Geometry: final body of the model. Coordinates: model frame, mm. Face numbers are marked on the shaded views. A direction names the side the tool comes from. Coordinates: 2 decimals unless noted, no trailing zeros. Write each loop counter-clockwise with the first axis right and the second up, starting at its lowest first coordinate (ties: lowest second). Pieces come first, ordered by that corner, then holes.
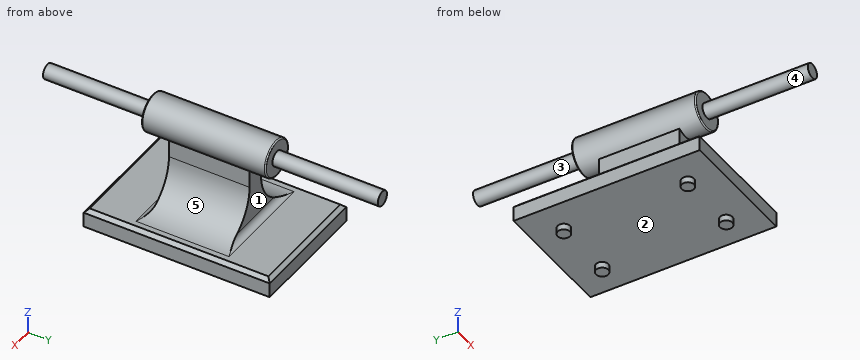
from build123d import *

# Parameters (mm, degrees)
F1_DEPTH  = 75
F2_W      = 15
F2_H      = 65
F3_DEPTH  = 70
F4_R      = 15
F5_DEPTH  = 50
F6_R      = 6
F7_DEPTH  = 85
F8_R      = 6
F9_DEPTH  = 85
F10_R     = 5
F11_DEPTH = 5
F12_R     = 35
F13_R     = 5
F14_SIZE  = 3
F15_R     = 1


with BuildPart() as f1:
    # F0 (on Front) → F1 (new body, symmetric)
    with BuildSketch(Plane.XZ):
        Polygon((50, -7.5), (50, 7.5), (-50, 7.5), (-50, -7.5), (-27.5, -7.5), (27.5, -7.5), align=None)
    extrude(amount=F1_DEPTH, both=True)

    # F2 (on Top) → F3 (join)
    with BuildSketch(Plane.XY):
        Rectangle(F2_W, F2_H)
    extrude(amount=F3_DEPTH)

    # F4 (on Front) → F5 (join, symmetric)
    with BuildSketch(Plane.XZ):
        with Locations((0, 69.991633)):
            Circle(F4_R)
    extrude(amount=F5_DEPTH, both=True)

    # F6 (on face) → F7 (join)
    with BuildSketch(Plane(origin=(0, 50, 0), x_dir=(-1, 0, 0), z_dir=(0, 1, 0))):
        with Locations((0, 69.991633)):
            Circle(F6_R)
    extrude(amount=F7_DEPTH)

    # F8 (on face) → F9 (join)
    with BuildSketch(Plane.XZ.offset(50)):
        with Locations((0, 69.991633)):
            Circle(F8_R)
    extrude(amount=F9_DEPTH)

    # F10 (on face) → F11 (join)
    with BuildSketch(Plane(origin=(0, 0, -7.5), x_dir=(1, 0, 0), z_dir=(0, 0, -1))):
        with Locations((-25, 50)):
            Circle(F10_R)
        with Locations((25, 50)):
            Circle(F10_R)
        with Locations((-25, -50)):
            Circle(F10_R)
        with Locations((25, -50)):
            Circle(F10_R)
    extrude(amount=F11_DEPTH)

    # F12
    f12_edges = [f1.edges().sort_by_distance(p)[0] for p in [
        (7.5, 0, 7.5),
        (-7.5, 0, 7.5),
    ]]
    fillet(f12_edges, radius=F12_R)

    # F13
    f13_edges = [f1.edges().sort_by_distance(p)[0] for p in [
        (25, -32.5, 7.5),
        (0, -32.5, 7.5),
        (-25, -32.5, 7.5),
        (25, 32.5, 7.5),
        (0, 32.5, 7.5),
        (-25, 32.5, 7.5),
    ]]
    fillet(f13_edges, radius=F13_R)

    # F14
    f14_edges = [f1.edges().sort_by_distance(p)[0] for p in [
        (-50, 0, 7.5),
        (0, 75, 7.5),
        (50, 0, 7.5),
        (0, -75, 7.5),
    ]]
    chamfer(f14_edges, length=F14_SIZE)

    # F15
    f15_edges = [f1.edges().sort_by_distance(p)[0] for p in [
        (-15, -50, 69.991633),
        (-15, 50, 69.991633),
    ]]
    fillet(f15_edges, radius=F15_R)


solid = f1.part
Item 1: Set-up query: the marked faces 3, 4 and 5. Return all of +Z, -Z, +X, -X, +Y, -Y with unobstructed straight access to the full face (end or side cutting, diameter ignored); none if empty.
Derived:
face 3: +Y
face 4: -Y
face 5: +X, +Y, -Y
Item 2: Material intervals for probe 1 along Z at (x, y) = (43.5, 8); probe 2 along Y at (x, z) = (-2.5, 22.5); probe 3 along Z at (x, y) = (0.5, 4), sorted ascending.
Derived:
probe 1: z = -7.5 to 7.5
probe 2: y = -32.5 to 32.5
probe 3: z = -7.5 to 84.98
Item 3: Pull-direction query (Z, two-part tool) for the marked faces 1 and 2; classes: released by +Z, released by -Z, zero draft, split by the parting line, or undercut.
Derived:
face 1: undercut
face 2: released by -Z
Item 4: Section B-B, the plane y = 25. Output: boundary loops of the cut face in (x, z), plus the area to 3 significant figures.
Derived:
outline: (-50, -7.5) - (50, -7.5) - (50, 4.5) - (47, 7.5) - (42.5, 7.5) arc R35 cw to (7.5, 42.5) - (7.5, 57) arc R15 ccw (long way) to (-7.5, 57) - (-7.5, 42.5) arc R35 cw to (-42.5, 7.5) - (-47, 7.5) - (-50, 4.5) - close
area: 3,450 mm2
Item 5: Section C-C, the plane z = 51.5. Output: boundary loops of the cut face in (x, y), plus the area to 3 significant figures.
Derived:
outline: (-7.5, -32.5) - (7.5, -32.5) - (7.5, 32.5) - (-7.5, 32.5) - close
area: 975 mm2
Item 6: Section A-A, the plane x = 0. Output: boundary loops of the cut face in (y, z).
Derived:
outline: (-135, 63.99) - (-50, 63.99) - (-50, 55.99) arc R1 ccw to (-49, 54.99) - (-32.5, 54.99) - (-32.5, 12.5) arc R5 cw to (-37.5, 7.5) - (-72, 7.5) - (-75, 4.5) - (-75, -7.5) - (75, -7.5) - (75, 4.5) - (72, 7.5) - (37.5, 7.5) arc R5 cw to (32.5, 12.5) - (32.5, 54.99) - (49, 54.99) arc R1 ccw to (50, 55.99) - (50, 63.99) - (135, 63.99) - (135, 75.99) - (50, 75.99) - (50, 83.99) arc R1 ccw to (49, 84.99) - (-49, 84.99) arc R1 ccw to (-50, 83.99) - (-50, 75.99) - (-135, 75.99) - close
Item 7: Pin query (flat end, axial travel): pin 1 (11.5 mm diameter, centred on y = 3.5, z = 51.5, fed in from -X); pin 2 (11.5 mm diameter, centred on y = -6.5, z = 52, fed in from +X); pin 3 (13.5 mm diameter, centred on x = -7.5, z = 44, fed in from -Y); pin 4 (14 mm diameter, centred on x = -1, z = 76, fed in from +Y). Return the tip coordinate at first contact, or that it passes through.
Derived:
pin 1: stops at x = -7.92
pin 2: stops at x = 8.67
pin 3: stops at y = -32.5
pin 4: stops at y = 135
Item 8: Section D-D, the plane x = 27. Output: boundary loops of the cut face in (y, z), plus the area to 3 significant figures.
Derived:
outline: (-75, -7.5) - (-54.58, -7.5) - (-54.58, -12.5) - (-45.42, -12.5) - (-45.42, -7.5) - (45.42, -7.5) - (45.42, -12.5) - (54.58, -12.5) - (54.58, -7.5) - (75, -7.5) - (75, 4.5) - (72, 7.5) - (37.5, 7.5) arc R5 cw to (32.69, 11.12) - (-32.69, 11.12) arc R5 cw to (-37.5, 7.5) - (-72, 7.5) - (-75, 4.5) - close
area: 2,580 mm2
